Design review of the part built by this model. Coordinates are the model's own, in mm. Face numbers are marked on the shaded views. Coordinates: 2 decimals unless noted, no trailing zeros. Order: outer loops, then holes, each group sorted by start corner. A loop starts at its lowest first (then second) coordinate and runs counter-clockwise, first axis right, second up. Notation, with made-up numbers: M 0.5,45 L 10.5,45 A8 cw 10.5,49 Z; hole C 46,-34.5 d7. An arc over 180 degrees is marked long. Answer as a JSON object with one key per item and string values.
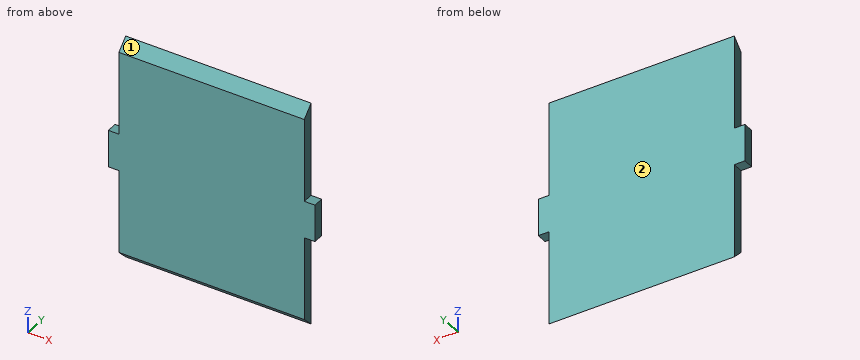
from build123d import *

# Parameters (mm, degrees)
SKETCH1_W           = 2
SKETCH1_H           = 7
SKETCH1_W_2         = 35
SKETCH1_H_2         = 42.42640687
BOSS_EXTRUDE1_DEPTH = 2
CUT_EXTRUDE1_DEPTH  = 43.995801746


with BuildPart() as part:
    # Sketch1 → Boss-Extrude1 (new body)
    with BuildSketch(Plane(origin=(0, 0, 0), x_dir=(1, 0, 0), z_dir=(0, 1, 0))):
        with Locations((-7.400304625, 0.597741848)):
            Rectangle(SKETCH1_W, SKETCH1_H)
        with Locations((11.099695375, 0.595945283)):
            Rectangle(SKETCH1_W_2, SKETCH1_H_2)
        with Locations((29.599695375, 0.597741848)):
            Rectangle(SKETCH1_W, SKETCH1_H)
    extrude(amount=BOSS_EXTRUDE1_DEPTH)

    # Sketch2 → Cut-Extrude1 (cut, through all)
    with BuildSketch(Plane(origin=(28.599695375, 0, 0), x_dir=(0, 0, -1), z_dir=(1, 0, 0))):
        Polygon((-20.617258152, 2), (-18.617258152, 0), (-20.617258152, 0), align=None)
        Polygon((21.809148718, 2), (21.809148718, 0), (19.809148718, 0), align=None)
    extrude(amount=-CUT_EXTRUDE1_DEPTH, mode=Mode.SUBTRACT)


solid = part.part
1) Add section B-B (z = 12). State the section outline as (x, y) points, and give its area (3 significant figures).
Taken from the geometry:
{"outline": "M -6.4,0 L 28.6,0 L 28.6,2 L -6.4,2 Z", "area": "70.0 mm2"}
2) Add section C-C (x = 13). State the section outline as (y, z) points, and give its area (3 significant figures).
Taken from the geometry:
{"outline": "M 0,-19.81 L 2,-21.81 L 2,20.62 L 0,18.62 Z", "area": "80.9 mm2"}
3) Insertion check: pin 1 Ø0.6 at (y, z) = (1.5, -17.5) entering from +X; pin 2 Ø0.6 at (y, z) = (0.5, 14.5) entering from -X; pin 3 Ø0.6 at (x, y) = (-8, 1) entering from -Z. Each pin has a flat end and moves straight along its axis. Give the tip position at first contact, or say it passes through.
Taken from the geometry:
{"pin 1": "stops at x = 28.6", "pin 2": "stops at x = -6.4", "pin 3": "stops at z = -4.1"}
4) Add section A-A (y = 1.5). State the section outline as (x, z) points.
Taken from the geometry:
{"outline": "M -8.4,-4.1 L -6.4,-4.1 L -6.4,-21.31 L 28.6,-21.31 L 28.6,-4.1 L 30.6,-4.1 L 30.6,2.9 L 28.6,2.9 L 28.6,20.12 L -6.4,20.12 L -6.4,2.9 L -8.4,2.9 Z"}
5) Mouldability with a two-part tool opening along Z and no side actions: class the marked faces 1 and 2 as released by +Z, released by -Z, zero draft, split by the parting line, or undercut.
Taken from the geometry:
{"face 1": "released by +Z", "face 2": "zero draft"}
6) To check wall thickness, follow L1, parallel to X at y = 1.3, z = -16.5; L2, parallel to Z at x = 3.5, y = 0.2; L3, parallel to Z at x = 1.5, y = 1.5. State the ranges of each line that lie inside material, in increasing order.
Taken from the geometry:
{"L1": "x = -6.4 to 28.6", "L2": "z = -20.01 to 18.82", "L3": "z = -21.31 to 20.12"}
